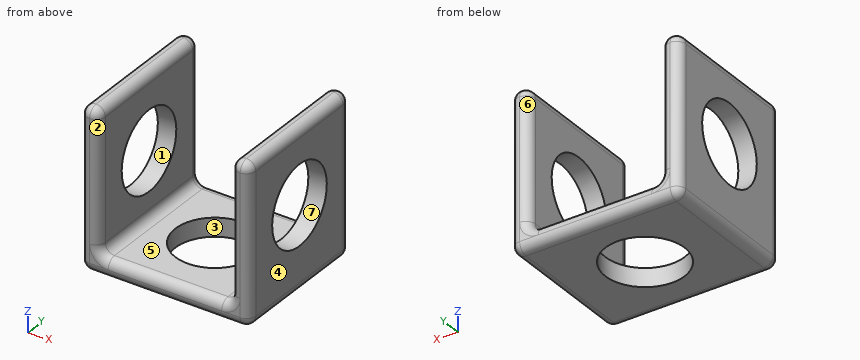
from build123d import *

# Parameters (mm, degrees)
SKETCH1_W           = 128
SKETCH1_H           = 120
BOSS_EXTRUDE1_DEPTH = 110
SKETCH2_W           = 100
SKETCH2_H           = 106
CUT_EXTRUDE2_DEPTH  = 208.084523806
SKETCH3_R           = 30
CUT_EXTRUDE3_DEPTH  = 208.084523806
SKETCH4_R           = 30
CUT_EXTRUDE4_DEPTH  = 200.298770694
FILLET1_R           = 7


with BuildPart() as part:
    # Sketch1 → Boss-Extrude1 (new body)
    with BuildSketch(Plane(origin=(0, 0, 0), x_dir=(1, 0, 0), z_dir=(0, 1, 0))):
        with Locations((64, 60)):
            Rectangle(SKETCH1_W, SKETCH1_H)
    extrude(amount=BOSS_EXTRUDE1_DEPTH)

    # Sketch2 → Cut-Extrude2 (cut, through all)
    with BuildSketch(Plane(origin=(0, 110, 0), x_dir=(1, 0, 0), z_dir=(0, 1, 0))):
        with Locations((64, 53)):
            Rectangle(SKETCH2_W, SKETCH2_H)
    extrude(amount=-CUT_EXTRUDE2_DEPTH, mode=Mode.SUBTRACT)

    # Sketch3 → Cut-Extrude3 (cut, through all)
    with BuildSketch(Plane.ZY):
        with Locations((-56, 55)):
            Circle(SKETCH3_R)
    extrude(amount=-CUT_EXTRUDE3_DEPTH, mode=Mode.SUBTRACT)

    # Sketch4 → Cut-Extrude4 (cut, through all)
    with BuildSketch(Plane.XY.offset(-106)):
        with Locations((64, 55)):
            Circle(SKETCH4_R)
    extrude(amount=-CUT_EXTRUDE4_DEPTH, mode=Mode.SUBTRACT)

    # Fillet1
    fillet1_edges = [part.edges().sort_by_distance(p)[0] for p in [
        (128, 110, -60),
        (121, 0, 0),
        (64, 110, -120),
        (121, 110, 0),
        (114, 55, 0),
        (14, 0, -53),
        (14, 55, 0),
        (64, 0, -106),
        (14, 55, -106),
        (114, 0, -53),
        (114, 55, -106),
        (114, 110, -53),
        (64, 110, -106),
        (14, 110, -53),
        (0, 110, -60),
        (64, 0, -120),
        (128, 0, -60),
        (7, 0, 0),
        (0, 0, -60),
        (0, 55, -120),
        (128, 55, -120),
        (128, 55, 0),
        (0, 55, 0),
        (7, 110, 0),
    ]]
    fillet(fillet1_edges, radius=FILLET1_R - 0.0001)  # a hair under: the kernel refuses the full size


solid = part.part
CAD build for the part. Positions are in the model's coordinates, mm. Face numbers are marked on the shaded views. A direction names the side the tool comes from. Coordinates: 2 decimals unless noted, no trailing zeros. Write item = value, one per line. Start each with the question number.
Q1. Pull direction Y, two halves, no side cores. Call the marked faces 1, 2, 3 and 4: pulls with the +Y half, pulls with the -Y half, needs draft (parallel to the pull), parting line crosses it, or undercut.
Q2. Cut at B-B, the plane y = 55. Give the number of separate pieces and of enclosed holes in the cut face, then the cut area to 3 significant figures.
Q3. Flat gauge pins, fed straight in: pin 1 Ø5 at (x, y) = (41, 85) entering from +Z; pin 2 Ø8 at (y, z) = (76.5, -49.5) entering from -X. Where does each tip first touch, or does it go through?
Q4. Which spindle directions (+Z, -Z, +X, -X, +Y, -Y) get a long thin tool onto all of the face, cutting with end or side? Do the marked faces 5, 6 and 7. Say none if no direction does.
Q5. Drill centre lines: L1, parallel to X at y = 86.5, z = -59.5; L2, parallel to Y at x = 121, z = -56; L3, parallel to Y at x = 10, z = -107.5. Where is each one in solid material? Low to high.
Computed:
q1.face_1 = undercut
q1.face_2 = pulls with the -Y half
q1.face_3 = undercut
q1.face_4 = needs draft
q2.separate_pieces = 4
q2.enclosed_holes = 0
q2.area = 2,200 mm²
q3.pin_1 = -106
q3.pin_2 = through
q4.face_5 = +Z, +Y, -Y
q4.face_6 = +Z, +Y
q4.face_7 = +X, -X
q5.L1 = 0 to 14, 114 to 128
q5.L2 = 0 to 25, 85 to 110
q5.L3 = 0 to 110
